from build123d import *

# Parameters (mm, degrees)
SKETCH1_W           = 62
SKETCH1_H           = 5.9
BOSS_EXTRUDE1_DEPTH = 8.1
SKETCH4_R           = 2.365
BOSS_EXTRUDE2_DEPTH = 3


with BuildPart() as part:
    # Sketch1 → Boss-Extrude1 (new body)
    with BuildSketch(Plane.XY):
        with Locations((0, 2.95)):
            Rectangle(SKETCH1_W, SKETCH1_H)
    extrude(amount=-BOSS_EXTRUDE1_DEPTH)

    # Sketch4 → Boss-Extrude2 (add)
    with BuildSketch(Plane(origin=(0, 0, -8.1), x_dir=(-1, 0, 0), z_dir=(0, 0, -1))):
        with Locations((23.8, 2.95)):
            Circle(SKETCH4_R)
    extrude(amount=BOSS_EXTRUDE2_DEPTH)


solid = part.part
The model under review builds one solid part; all positions refer to its coordinate system, in mm. A direction names the side the tool comes from. Give positions to 0.01 mm unless a question says otherwise; leave off trailing zeros. Order: outer loops, then holes, each group sorted by start corner. A loop starts at its lowest first (then second) coordinate and runs counter-clockwise, first axis right, second up. Notation, with made-up numbers: M 50.25,82.25 L 104.25,82.25 A29 cw 104.25,113.25 Z; hole C 65.25,1.5 d1. An arc over 180 degrees is marked long. One line per question, with ' | ' between items. Start each with the question number.
1) Wall thickness on L1, parallel to Z at x = 11, y = 5.5; L2, parallel to X at y = 4.9, z = -9.75: over which ranges is each line inside the solid? List them lowest first. Write a range as from..to.
2) Consider section C-C, the plane x = -14.5. Give the boundary of the cut face in (y, z).
3) Consider section A-A, the plane x = -23.8. Give the boundary of the cut face in (y, z) (3 decimals).
4) Consider section B-B, the plane y = 4.4. Give the boundary of the cut face in (x, z).
5) For faces 1 (the face through (-25.985, 2.044, -9.579)), 2 (the face through (31, 3, -4)), list the 3-axis set-ups (+Z, -Z, +X, -X, +Y, -Y) from which the entire face can be reached by the end or side of a thin tool; tool diameter is ignored.
Found:
1) L1: z = -8.1..0 | L2: x = -25.14..-22.46
2) outline: M 0,-8.1 L 5.9,-8.1 L 5.9,0 L 0,0 Z
3) outline: M 0,-8.1 L 0.585,-8.1 L 0.585,-11.1 L 5.315,-11.1 L 5.315,-8.1 L 5.9,-8.1 L 5.9,0 L 0,0 Z
4) outline: M -31,-8.1 L -25.67,-8.1 L -25.67,-11.1 L -21.93,-11.1 L -21.93,-8.1 L 31,-8.1 L 31,0 L -31,0 Z
5) face 1: -Z | face 2: +Z, -Z, +X, +Y, -Y
